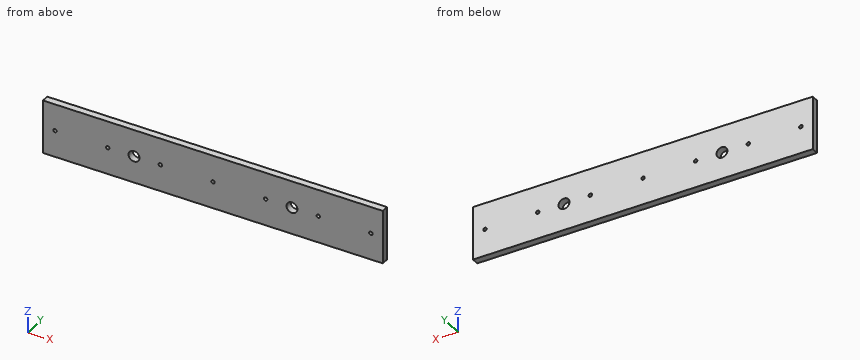
```python
from build123d import *

# Parameters (mm, degrees)
CROQUIS1_W              = 310
CROQUIS1_H              = 50
SALIENTE_EXTRUIR1_DEPTH = 6.35
CROQUIS2_R              = 1.5875
CROQUIS2_R_2            = 5
CORTAR_EXTRUIR3_DEPTH   = 7.35


with BuildPart() as part:
    # Croquis1 → Saliente-Extruir1 (new body)
    with BuildSketch(Plane(origin=(0, 0, 0), x_dir=(1, 0, 0), z_dir=(0, 1, 0))):
        Rectangle(CROQUIS1_W, CROQUIS1_H)
    extrude(amount=SALIENTE_EXTRUIR1_DEPTH)

    # Croquis2 → Cortar-Extruir3 (cut, through all)
    with BuildSketch(Plane(origin=(0, 6.35, 0), x_dir=(1, 0, 0), z_dir=(0, 1, 0))):
        Circle(CROQUIS2_R)
        with Locations((-144, 0)):
            Circle(CROQUIS2_R)
        with Locations((144, 0)):
            Circle(CROQUIS2_R)
        with Locations((48, 0)):
            Circle(CROQUIS2_R)
        with Locations((96, 0)):
            Circle(CROQUIS2_R)
        with Locations((-48, 0)):
            Circle(CROQUIS2_R)
        with Locations((-96, 0)):
            Circle(CROQUIS2_R)
        with Locations((-72, 0)):
            Circle(CROQUIS2_R_2)
        with Locations((72, 0)):
            Circle(CROQUIS2_R_2)
    extrude(amount=-CORTAR_EXTRUIR3_DEPTH, mode=Mode.SUBTRACT)


solid = part.part
```
The model under review builds one solid part; all positions refer to its coordinate system, in mm. Give positions to 0.01 mm unless a question says otherwise; leave off trailing zeros. Write each loop counter-clockwise with the first axis right and the second up, starting at its lowest first coordinate (ties: lowest second). Pieces come first, ordered by that corner, then holes. Notation, with made-up numbers: (-12.5, 70) -> (41.5, 70) arc R36 cw to (41.5, 106) -> close; hole circle Ø3 at (-4, 88). An arc over 180 degrees is marked (long way). Answer in a Markdown table with one row per item.
1) For L1, parallel to Z at x = 48, y = 3.75; L2, parallel to Z at x = 72, y = 5.25, list the stretches that pass through material, from the lowest coordinate up. Write a range as [from, to].
Worked answers:
| item | result |
|---|---|
| L1 | [-25, -1.59], [1.59, 25] |
| L2 | [-25, -5], [5, 25] |
2) Clearance check with a flat-ended pin moving along its axis: P1, Ø2.5, axis at x = -144, z = 0, coming from the +Y side. State where the tip first meets the part, or that it passes through.
Worked answers:
| item | result |
|---|---|
| P1 | through |
3) Add section A-A on x = 72. State the section outline as (y, z) points, plus the area to 3 significant figures.
Worked answers:
| item | result |
|---|---|
| outline | (0, -25) -> (6.35, -25) -> (6.35, -5) -> (0, -5) -> close; (0, 5) -> (6.35, 5) -> (6.35, 25) -> (0, 25) -> close |
| area | 254 mm² |
